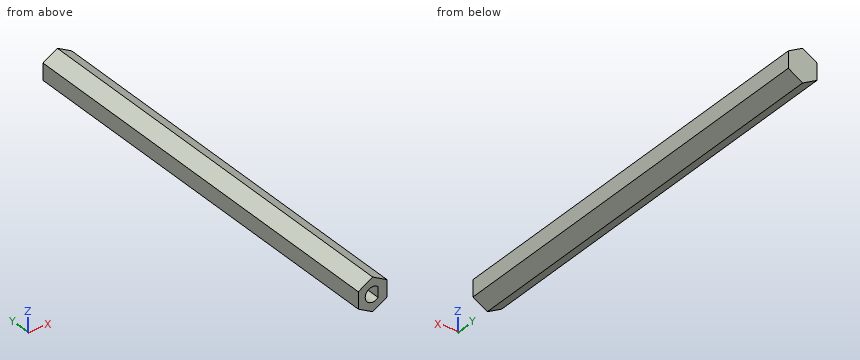
```python
from build123d import *

# Parameters (mm, degrees)
BOSS_EXTRUDE1_DEPTH = 151.892
CUT_EXTRUDE1_DEPTH  = 10.16


with BuildPart() as part:
    # Sketch1 → Boss-Extrude1 (new body)
    with BuildSketch(Plane(origin=(0, 0, 0), x_dir=(1, 0, 0), z_dir=(0, 1, 0))):
        Polygon((-5.279290861, -3.048), (0, -6.096), (5.279290861, -3.048), (5.279290861, 3.048), (0, 6.096), (-5.279290861, 3.048), align=None)
    extrude(amount=BOSS_EXTRUDE1_DEPTH)

    # Sketch1_3 → Cut-Extrude1 (cut)
    with BuildSketch(Plane(origin=(0, 0, 0), x_dir=(1, 0, 0), z_dir=(0, 1, 0))):
        with BuildLine():
            Line((2, -1.858932557), (2, 1.858932557))
            ThreePointArc((2, 1.858932557), (-2.7305, 0), (2, -1.858932557))
        make_face()
    extrude(amount=CUT_EXTRUDE1_DEPTH, mode=Mode.SUBTRACT)


solid = part.part
```
Design review of the part built by this model. Coordinates are the model's own, in mm. Round coordinates to 2 decimals unless told otherwise and drop trailing zeros. Order: outer loops, then holes, each group sorted by start corner. A loop starts at its lowest first (then second) coordinate and runs counter-clockwise, first axis right, second up. Notation, with made-up numbers: (-24.75, -28) - (30.25, -28) arc R29 cw to (30.25, -2) - close; hole circle Ø2 at (41.25, -10). An arc over 180 degrees is marked (long way). Return JSON: item names as keys, results as strings.
Q1. Consider section A-A on z = 0. Write out the cut boundary in (x, y).
Computed values:
{"outline": "(-5.28, 0) - (-2.73, 0) - (-2.73, 10.16) - (2, 10.16) - (2, 0) - (5.28, 0) - (5.28, 151.89) - (-5.28, 151.89) - close"}
Q2. Wall thickness on L1, parallel to X at y = 5.25, z = 0; L2, parallel to Z at x = 0, y = 5.75; L3, parallel to Y at x = 1.25, z = 1.5: over which ranges is each line inside the solid? List them lowest first. Write a range as [from, to].
Computed values:
{"L1": "x = [-5.28, -2.73], [2, 5.28]", "L2": "z = [-6.1, -2.73], [2.73, 6.1]", "L3": "y = [10.16, 151.89]"}
Q3. Consider section C-C on x = -4. Write out the cut boundary in (y, z).
Computed values:
{"outline": "(0, -3.79) - (151.89, -3.79) - (151.89, 3.79) - (0, 3.79) - close"}
Q4. Consider section B-B on y = 112. Write out the cut boundary in (x, z).
Computed values:
{"outline": "(-5.28, -3.05) - (0, -6.1) - (5.28, -3.05) - (5.28, 3.05) - (0, 6.1) - (-5.28, 3.05) - close"}
Q5. For pin 1 Ø6 at (y, z) = (85.5, 4) entering from +X; pin 2 Ø1.5 at (y, z) = (121.5, -4) entering from -X; pin 3 Ø4 at (x, y) = (-2.5, 135) entering from -Z, all flat-tipped, find the tip position at first contact; note any pin that passes through.
Computed values:
{"pin 1": "stops at x = 5.28", "pin 2": "stops at x = -4.93", "pin 3": "stops at z = -5.81"}
